Source: three-view drawing plus pictorial views. Frame: mm from the lowest corner of the part. Round coordinates to 2 decimals unless told otherwise and drop trailing zeros. Order: outer loops, then holes, each group sorted by start corner. A loop starts at its lowest first (then second) coordinate and runs counter-clockwise, first axis right, second up. Notation, with made-up numbers: (87.25, 14.25) - (105.25, 14.25) arc R19 ccw to (105.25, 38.25) - close; hole circle Ø5 at (1, 69.25). An arc over 180 degrees is marked (long way). Use one line per item in the form item = value. Start each with the question number.
Q1. Cut plane D-D, the plane x = 34. Return the cut outline in (y, z), and give its area (3 significant figures).
Q2. Draft query along Z for the marked faces 1 and 2. Return one class per face: released by +Z, released by -Z, zero draft, split by the parting line, or undercut.
Q3. Cut plane C-C, the plane x = 25.5. Return the cut outline in (y, z).
Q4. Cut plane A-A, the plane y = 1.8. Return the cut outline in (x, z).
Q5. Cut plane B-B, the plane z = 1.5. Return the cut outline in (x, y), and give its area (3 significant figures).
Q6. Ray query, line 1 (X direction, y = 1.6, z = 1.5); line 2 (Z direction, x = 34, y = 1.9); line 3 (X direction, y = 2.1, z = 9.5). Return the intervals inside material, ascending. Write a range as [from, to].
Q7. Pin query (flat end, axial travel): pin 1 Ø2 at (x, z) = (19, 11) entering from +Y. Return the tip coordinate at first contact, or that it passes through.
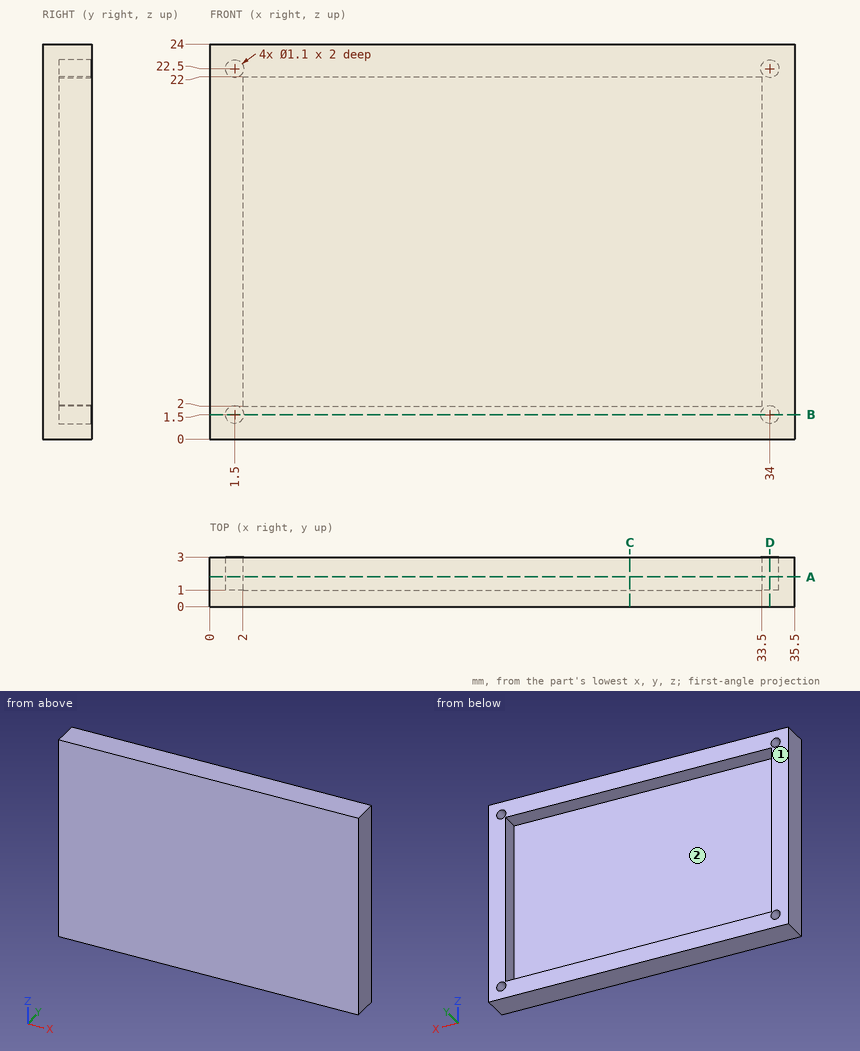
Completed:
q1.outline = (0, 0) - (3, 0) - (3, 0.95) - (1, 0.95) - (1, 2.05) - (3, 2.05) - (3, 21.95) - (1, 21.95) - (1, 23.05) - (3, 23.05) - (3, 24) - (0, 24) - close
q1.area = 67.6 mm2
q2.face_1 = zero draft
q2.face_2 = undercut
q3.outline = (0, 0) - (3, 0) - (3, 2) - (1, 2) - (1, 22) - (3, 22) - (3, 24) - (0, 24) - close
q4.outline = (0, 0) - (35.5, 0) - (35.5, 24) - (0, 24) - close; hole circle Ø1.1 at (1.5, 1.5); hole circle Ø1.1 at (1.5, 22.5); hole (2, 2) - (33.5, 2) - (33.5, 22) - (2, 22) - close; hole circle Ø1.1 at (34, 1.5); hole circle Ø1.1 at (34, 22.5)
q5.outline = (0, 0) - (35.5, 0) - (35.5, 3) - (34.55, 3) - (34.55, 1) - (33.45, 1) - (33.45, 3) - (2.05, 3) - (2.05, 1) - (0.95, 1) - (0.95, 3) - (0, 3) - close
q5.area = 102 mm2
q6.line_1 = [0, 0.95], [2.05, 33.45], [34.55, 35.5]
q6.line_2 = [0, 0.95], [2.05, 21.95], [23.05, 24]
q6.line_3 = [0, 2], [33.5, 35.5]
q7.pin_1 = 1
